The figure shows three views and two pictorial views of one solid part (mm, origin at its lowest corner). Answer the questions. Give positions to 0.01 mm unless a question says otherwise; leave off trailing zeros. Order: outer loops, then holes, each group sorted by start corner. A loop starts at its lowest first (then second) coordinate and runs counter-clockwise, first axis right, second up. Notation, with made-up numbers: (47.25, -0.5) - (88.25, -0.5) arc R22 ccw to (88.25, 33.5) - close; hole circle Ø9 at (12, 15). An arc over 180 degrees is marked (long way). Answer as CSV lines item,"result". Start each with the question number.
1. Section B-B on y = 6.75 is taken. Give the vertices of the cut face in (x, z) (3 decimals).
2. Section D-D on x = 108 is taken. Give the vertices of the cut face in (y, z).
3. Flat-ended cylindrical pins translate along their axes: pin 1 (8 mm diameter, centred on y = 20.5, z = 220, fed in from -X); pin 2 (10 mm diameter, centred on y = 3.5, z = 169, fed in from +X) (3 decimals). Find the tip coordinate at first contact, or state that the pin passes through.
4. Consider line 1 along Z through (x, y) = (142.5, 17.5); line 2 along Z through (x, y) = (70.5, 1.75); line 3 along X through (y, z) = (20.75, 343.5) (3 decimals). Determine where each line is inside the solid, lowest interval first. Write a range as [from, to].
5. Section A-A on x = 63.5 is taken. Give the vertices of the cut face in (y, z), and give its area (3 significant figures).
6. Section C-C on z = 185 is taken. Give the vertices of the cut face in (x, y) (3 decimals), and give its area (3 significant figures).
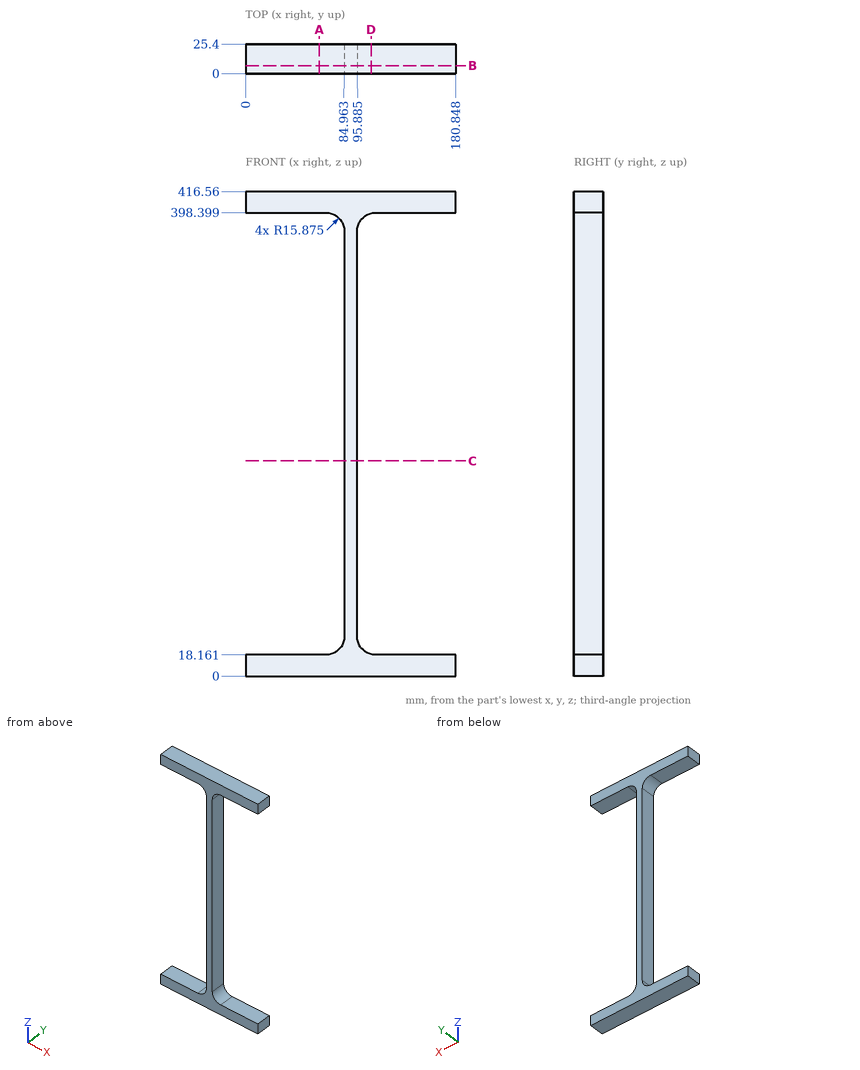
Checks:
1,outline,"(0, 0) - (180.848, 0) - (180.848, 18.161) - (111.76, 18.161) arc R15.875 cw to (95.885, 34.036) - (95.885, 382.524) arc R15.875 cw to (111.76, 398.399) - (180.848, 398.399) - (180.848, 416.56) - (0, 416.56) - (0, 398.399) - (69.088, 398.399) arc R15.875 cw to (84.963, 382.524) - (84.963, 34.036) arc R15.875 cw to (69.088, 18.161) - (0, 18.161) - close"
2,outline,"(0, 0) - (25.4, 0) - (25.4, 18.61) - (0, 18.61) - close; (0, 397.95) - (25.4, 397.95) - (25.4, 416.56) - (0, 416.56) - close"
3,pin 1,"stops at x = 84.96"
3,pin 2,"stops at x = 95.885"
4,line 1,"z = [0, 18.16], [398.4, 416.56]"
4,line 2,"z = [0, 18.22], [398.34, 416.56]"
4,line 3,"x = [84.963, 95.885]"
5,outline,"(0, 0) - (25.4, 0) - (25.4, 18.16) - (0, 18.16) - close; (0, 398.4) - (25.4, 398.4) - (25.4, 416.56) - (0, 416.56) - close"
5,area,"923 mm²"
6,outline,"(84.963, 0) - (95.885, 0) - (95.885, 25.4) - (84.963, 25.4) - close"
6,area,"277 mm²"
